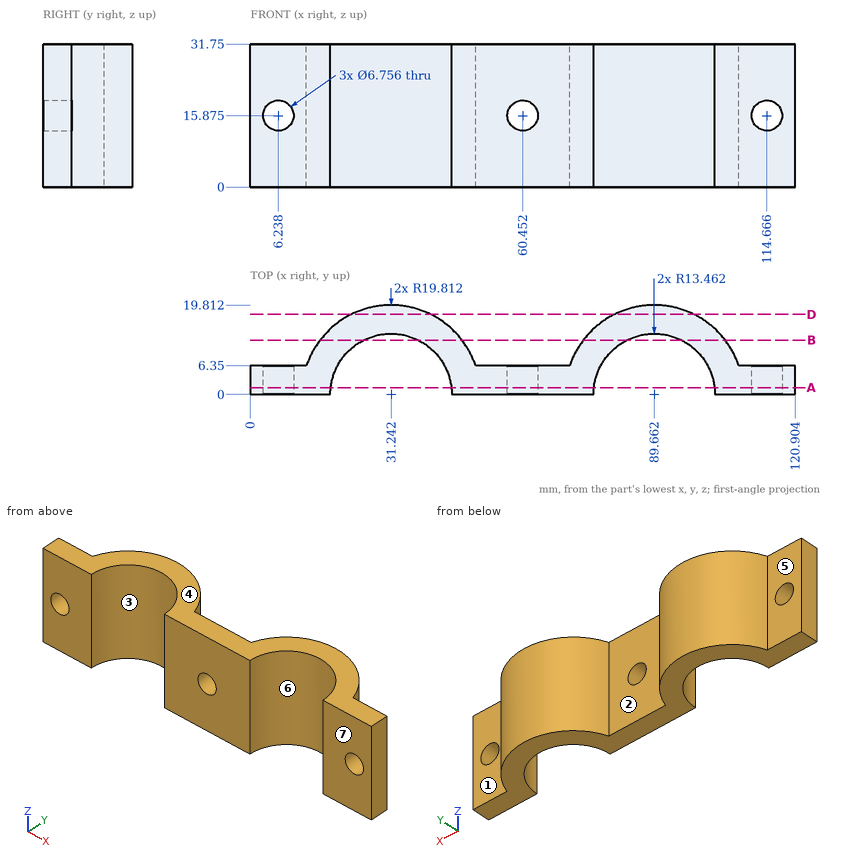
The drawing under review shows one solid part. Ordinate dimensions are in mm from its lowest x, y, z. A direction names the side the tool comes from. Coordinates: 2 decimals unless noted, no trailing zeros. Write each loop counter-clockwise with the first axis right and the second up, starting at its lowest first coordinate (ties: lowest second). Pieces come first, ordered by that corner, then holes. Notation, with made-up numbers: (-28, 60) -> (17, 60) arc R23 ccw to (17, 72) -> close; hole circle Ø2 at (-33, 55.5). An arc over 180 degrees is marked (long way). One line per item, written item: value. Start each with the question number.
Q1. To check wall thickness, follow probe 1 along X at (y, z) = (11, 11) (1 decimal); probe 2 along X at (y, z) = (3, 20.5) (1 decimal); probe 3 along X at (y, z) = (10.25, 8.5) (1 decimal). State the ranges of each line that lie inside material, in increasing order.
Q2. The part is to be moulded in two halves that separate along X. For the marked faces 6 and 7, say which applies: +X half, -X half, draft (parallel to the pull), parting line (faces both ways), or undercut.
Q3. Clearance check with flat-ended pins moving along their axes: P1, Ø8, axis at y = 11, z = 9, coming from the +X side; P2, Ø8, axis at x = 6.24, z = 15.88, coming from the +Y side; P3, Ø13.5, axis at x = 113.5, z = 21.5, coming from the +Y side (1 decimal). State where each tip first meets the part, or that it passes through.
Q4. Add section A-A, the plane y = 1.5. Count the separate pieces of the cut face and the enclosed holes in it, then the cut area to 3 significant figures.
Q5. For the marked faces 1, 2, 3, 4 and 5, list the 3-axis set-ups (+Z, -Z, +X, -X, +Y, -Y) from which the entire face can be reached by the end or side of a thin tool; tool diameter is ignored.
Q6. Add section D-D, the plane y = 17.75. Give the boundary of the cut face in (x, z), then the cut area to 3 significant figures.
Q7. Add section B-B, the plane y = 12. Give the boundary of the cut face in (x, z), then the cut area to 3 significant figures.
Response:
1. probe 1: 14.8 to 23.5, 39 to 47.7, 73.2 to 81.9, 97.4 to 106.1
1. probe 2: 0 to 18.1, 44.4 to 76.5, 102.8 to 120.9
1. probe 3: 14.3 to 22.5, 40 to 48.2, 72.7 to 80.9, 98.4 to 106.6
2. face 6: undercut
2. face 7: draft
3. P1: x = 108.2
3. P2: y = 6.35
3. P3: y = 10
4. separate pieces: 3
4. enclosed holes: 3
4. area: 2,030 mm²
5. face 1: +Z, -Z, +X, +Y
5. face 2: +Z, -Z, +Y
5. face 3: +Z, -Z, -Y
5. face 4: +Z, +X, -X, +Y, -Y
5. face 5: +Z, -Z, -X, +Y
6. outline: (22.44, 0) -> (40.04, 0) -> (40.04, 31.75) -> (22.44, 31.75) -> close; (80.86, 0) -> (98.46, 0) -> (98.46, 31.75) -> (80.86, 31.75) -> close
6. area: 1,120 mm²
7. outline: (15.48, 0) -> (25.14, 0) -> (25.14, 31.75) -> (15.48, 31.75) -> close; (37.34, 0) -> (47.01, 0) -> (47.01, 31.75) -> (37.34, 31.75) -> close; (73.9, 0) -> (83.56, 0) -> (83.56, 31.75) -> (73.9, 31.75) -> close; (95.76, 0) -> (105.43, 0) -> (105.43, 31.75) -> (95.76, 31.75) -> close
7. area: 1,230 mm²
